from build123d import *

# Parameters (mm, degrees)
SKETCH1_R           = 55
BOSS_EXTRUDE1_DEPTH = 60
SKETCH2_R           = 42.5
BOSS_EXTRUDE2_DEPTH = 130
FILLET2_R           = 10
SKETCH3_R           = 42.5
CUT_EXTRUDE1_DEPTH  = 110


with BuildPart() as part:
    # Sketch1 → Boss-Extrude1 (new body, symmetric)
    with BuildSketch(Plane(origin=(0, 0, 0), x_dir=(1, 0, 0), z_dir=(0, 1, 0))):
        Circle(SKETCH1_R)
    extrude(amount=BOSS_EXTRUDE1_DEPTH, both=True)

    # Sketch2 → Boss-Extrude2 (add)
    with BuildSketch(Plane.XY):
        Circle(SKETCH2_R)
    extrude(amount=BOSS_EXTRUDE2_DEPTH)

    # Fillet2
    fillet2_edges = [part.edges().sort_by_distance(p)[0] for p in [
        (-55, -60, 0),
    ]]
    fillet(fillet2_edges, radius=FILLET2_R)

    # Sketch3 → Cut-Extrude1 (cut)
    with BuildSketch(Plane(origin=(0, 0, 0), x_dir=(1, 0, 0), z_dir=(0, 1, 0))):
        Circle(SKETCH3_R)
    extrude(amount=CUT_EXTRUDE1_DEPTH, mode=Mode.SUBTRACT)


solid = part.part
Design review of the part built by this model. Coordinates are the model's own, in mm. A direction names the side the tool comes from. Coordinates: 2 decimals unless noted, no trailing zeros. Loops run counter-clockwise (first coordinate to the right, second up) from the corner with the lowest first, then second, coordinate; pieces in that order, holes last. Notation, with made-up numbers: (32, 73.5) -> (63, 73.5) arc R6 cw to (63, 79.5) -> close; hole circle Ø4 at (55.25, 78). An arc over 180 degrees is marked (long way). Use a Markdown table: item, result. Add a question column.
Item 1: We need section C-C, the plane y = 35. Write out the cut boundary in (x, z), and give its area (3 significant figures).
Item 2: Clearance check with flat-ended pins moving along their axes: P1, Ø1, axis at x = 37.5, z = 50.5, coming from the -Y side; P2, Ø1, axis at x = -18, y = -43.5, coming from the +Z side; P3, Ø5, axis at x = 43, y = 8.5, coming from the -Z side. State where each tip first meets the part, or that it passes through.
Item 3: Machinability: for faces 1 (the flat face through (-1, -60, -1)), 2 (the flat face through (-1, 0, -1)), which of the approach directions +Z, -Z, +X, -X, +Y, -Y give a long, thin tool a straight path to every point of the face, cutting with its end or side? Answer none if there is none.
Item 4: The part is to be moulded in two halves that separate along Z. For faces 3 (the cylindrical face through (22.848, 35.836, 81.79)), 4 (the cylindrical face through (-33.727, 29.58, 25.861)), 5 (the cylindrical face through (-7.16, 5.77, -54.53)), say which applies: +Z half, -Z half, draft (parallel to the pull), parting line (faces both ways), or undercut.
Item 5: We need section A-A, the plane z = 0. Write out the cut boundary in (x, y).
Item 6: We need section D-D, the plane y = -47. Write out the cut boundary in (x, z), and give its area (3 significant figures).
Item 7: Wall thickness on L1, parallel to X at y = 36, z = 0; L2, parallel to Y at x = -15, z = 7; L3, parallel to Z at x = 0, y = 31: over which ranges is each line inside the solid? List them lowest first. Write a range as from..to.
Item 8: We need section B-B, the plane x = 0. Write out the cut boundary in (y, z).
Numbers:
| question | item | result |
|---|---|---|
| 1 | outline | (-24.11, 49.43) arc R55 ccw (long way) to (24.11, 49.43) -> (24.11, 130) -> (-24.11, 130) -> close; hole circle Ø85 at (0, 0) |
| 1 | area | 7,530 mm^2 |
| 2 | P1 | stops at y = -20.91 |
| 2 | P2 | stops at z = 52.14 |
| 2 | P3 | stops at z = -37.21 |
| 3 | face 1 | +Z, -Z, +X, -X, -Y |
| 3 | face 2 | +Y |
| 4 | face 3 | draft |
| 4 | face 4 | undercut |
| 4 | face 5 | parting line |
| 5 | outline | (-55, -50) arc R10 ccw to (-45, -60) -> (45, -60) arc R10 ccw to (55, -50) -> (55, 60) -> (42.5, 60) -> (42.5, 0) -> (-42.5, 0) -> (-42.5, 60) -> (-55, 60) -> close |
| 6 | outline | circle Ø110 at (0, 0) |
| 6 | area | 9,500 mm^2 |
| 7 | L1 | x = -55..-42.5, 42.5..55 |
| 7 | L2 | y = -60..0 |
| 7 | L3 | z = -55..-42.5, 42.5..130 |
| 8 | outline | (-60, -45) arc R10 ccw to (-50, -55) -> (60, -55) -> (60, -42.5) -> (0, -42.5) -> (0, 42.5) -> (60, 42.5) -> (60, 55) -> (42.5, 55) -> (42.5, 130) -> (-42.5, 130) -> (-42.5, 55) -> (-50, 55) arc R10 ccw to (-60, 45) -> close |
